Read the model definition and answer for the solid it produces. Units are mm, in the model's axes. A direction names the side the tool comes from. Give positions to 0.01 mm unless a question says otherwise; leave off trailing zeros. Order: outer loops, then holes, each group sorted by start corner. A loop starts at its lowest first (then second) coordinate and runs counter-clockwise, first axis right, second up. Notation, with made-up numbers: (45.25, 71.5) -> (104.25, 71.5) arc R19 ccw to (104.25, 81.5) -> close; hole circle Ø1 at (22, 19). An arc over 180 degrees is marked (long way). Use one line per item in the form item = value.
Autodesk Inventor part; units mm, degrees
ref_plane "YZ Plane" through (0, 0, 0) normal (1, 0, 0) x (0, 1, 0)
ref_plane "XZ Plane" through (0, 0, 0) normal (0, 1, 0) x (-1, 0, 0)
ref_plane "XY Plane" through (0, 0, 0) normal (0, 0, 1) x (1, 0, 0)
sketch "Sketch1" plane through (0, 0, 0) normal (1, 0, 0) x (0, 1, 0)
  line L0 (-7.5, 10.5) -> (7.5, 10.5)
  line L1 (7.5, 10.5) -> (7.5, -10.5)
  line L2 (7.5, -10.5) -> (-7.5, -10.5)
  line L3 (-7.5, -10.5) -> (-7.5, 10.5)
  point P0 (0, 0)
  dimension "d0" = 21
  dimension "d1" = 15
  dimension "d2" = 7.5
  dimension "d3" = 10.5
extrude "Extrusion1" add sketch "Sketch1" along normal blind 2
fillet "Fillet1" radius 1 4 edges at (1, -7.5, -10.5) (1, 7.5, -10.5) (1, 7.5, 10.5) (1, -7.5, 10.5)
sketch "Sketch2" plane through (2, 0, 0) normal (1, 0, 0) x (0, 0, -1)
  line L0 (-7.15, 4.85) -> (7.15, 4.85)
  line L1 (7.15, 4.85) -> (7.15, -4.85)
  line L2 (7.15, -4.85) -> (-7.15, -4.85)
  line L3 (-7.15, -4.85) -> (-7.15, 4.85)
  point P0 (0, 0)
  dimension "d7" = 4.85
  dimension "d8" = 9.7
  dimension "d9" = 14.3
  dimension "d10" = 7.15
ref_plane "Work Plane1" through (2, -4.85, 7.15) normal (0, -1, 0) x (1, 0, 0)
sketch "Sketch3" plane through (2, -4.85, 7.15) normal (0, -1, 0) x (1, 0, 0)
  arc A0 (3.5, -2.0473) -> (0, 0) centre (-3.3399, -9.7251) ccw
  line L0 (0, -16.65) -> (0, 2.35)
  arc A1 (3.5, -2.0473) -> (0, -14.3) centre (22.3145, -14.0479) ccw
  point P0 (-2, -7.15)
  point P1 (0, -13.7959)
  dimension "d11" = 3.5
extrude "Extrusion2" add sketch "Sketch3" against normal blind 9.7
sketch "Sketch4" plane through (0, 0, 0) normal (-1, 0, 0) x (0, 0, 1)
  line L0 (9.25, -6) -> (-9.25, -6)
  line L1 (-9.25, -6) -> (-9.25, 6)
  line L2 (-9.25, 6) -> (9.25, 6)
  line L3 (9.25, 6) -> (9.25, -6)
  line L4 (9.5, -7.5) -> (-9.5, -7.5)
  line L5 (10.5, 6.5) -> (10.5, -6.5)
  point P0 (0, 0)
  dimension "d14" = 18.5
  dimension "d15" = 12
  dimension "d16" = 1.5
  dimension "d17" = 1.25
extrude "Extrusion3" add sketch "Sketch4" along normal blind 12.3
sketch "Sketch5" plane through (-12.3, 0, 0) normal (-1, 0, 0) x (0, 0, 1)
  line L0 (9.25, -6) -> (9.25, 6)
  line L1 (-9.25, -6) -> (-9.25, 6)
  line L2 (9.25, 2.5) -> (-9.25, 2.5)
  line L3 (-9.25, 2.5) -> (-9.25, -2.5)
  line L4 (-9.25, -2.5) -> (9.25, -2.5)
  line L5 (9.25, -2.5) -> (9.25, 2.5)
  line L6 (9.25, 6) -> (-9.25, 6)
  point P0 (0, 0)
  point P1 (9.25, -2.5)
  point P2 (-9.25, 2.5)
  dimension "d20" = 5
  dimension "d21" = 3.5
extrude "Extrusion4" add sketch "Sketch5" along normal blind 6.2 contours L4 L1 L2 L0
sketch "Sketch6" plane through (-18.5, 0, 0) normal (-1, 0, 0) x (0, 0, 1)
  line L0 (9.25, 2.5) -> (-9.25, 2.5)
  line L1 (-9.25, 2.5) -> (-9.25, -2.5)
  line L2 (-9.25, -2.5) -> (9.25, -2.5)
  line L3 (9.25, -2.5) -> (9.25, 2.5)
  line L4 (9.25, 2.5) -> (8.25, 2.5)
  line L5 (8.25, 2.5) -> (8.25, -2.5)
  line L6 (8.25, -2.5) -> (9.25, -2.5)
  line L7 (9.25, -2.5) -> (9.25, 2.5)
  line L8 (7.25, -2.5) -> (0.75, -2.5)
  line L9 (0.75, -2.5) -> (0.75, 2.5)
  line L10 (0.75, 2.5) -> (7.25, 2.5)
  line L11 (7.25, 2.5) -> (7.25, -2.5)
  line L12 (-9.25, 2.5) -> (9.25, 2.5)
  line L13 (-7.25, -2.5) -> (-0.25, -2.5)
  line L14 (-0.25, -2.5) -> (-0.25, 2.5)
  line L15 (-0.25, 2.5) -> (-7.25, 2.5)
  line L16 (-7.25, 2.5) -> (-7.25, -2.5)
  line L17 (9.25, -2.5) -> (-9.25, -2.5)
  line L18 (-9.25, 2.5) -> (-8.25, 2.5)
  line L19 (-8.25, 2.5) -> (-8.25, -2.5)
  line L20 (-8.25, -2.5) -> (-9.25, -2.5)
  line L21 (-9.25, -2.5) -> (-9.25, 2.5)
  point P0 (0, 0)
  point P1 (-8.25, -2.5)
  point P2 (-0.25, -2.5)
  point P3 (7.25, 2.5)
  dimension "d24" = 1
  dimension "d25" = 1
  dimension "d26" = 1
  dimension "d27" = 1
  dimension "d28" = 1
  dimension "d29" = 6.5
extrude "Extrusion5" cut sketch "Sketch6" against normal blind 6.2 contours L3 L2 L5 L0 | L11 L2 L9 L0 | L14 L2 L16 L0 | L19 L2 L1 L0
chamfer "Chamfer1" distance 1.5 angle 45 6 edges at (-18.5, 2.5, -7.75) (-18.5, -2.5, -7.75) (-18.5, -2.5, 0.25) (-18.5, 2.5, 0.25) (-18.5, -2.5, 7.75) (-18.5, 2.5, 7.75)
sketch "Sketch7" plane through (-12.3, -2.5, -8.25) normal (0, 0, -1) x (-1, 0, 0)
  line L0 (6.2, 1.5) -> (4.7, 0)
  line L1 (6.2, 3.5) -> (6.2, 1.5)
  line L2 (4.7, 5) -> (6.2, 3.5)
  line L3 (0, 5) -> (4.7, 5)
  line L4 (0, 5) -> (0, 0)
  line L5 (4.7, 0) -> (0, 0)
  point P0 (-12.3, 2.5)
  point P1 (5.2, 2.5)
  point P2 (4.1377, 2.5)
hole "Hole1" at (-16.4377, 0, -8.25) direction (0, 0, 1) diameter 2.2 end through all
sketch "Sketch8" plane through (0, 0, 0) normal (-1, 0, 0) x (0, 0, 1)
  line L0 (-9.7, -6.55) -> (9.7, -6.55)
  line L1 (9.7, -6.55) -> (9.7, 6.55)
  line L2 (9.7, 6.55) -> (-9.7, 6.55)
  line L3 (-9.7, 6.55) -> (-9.7, -6.55)
  line L4 (-9.7, -6.55) -> (9.7, 6.55) construction
  line L5 (9.7, -6.55) -> (-9.7, 6.55) construction
  point P0 (0, 0)
  dimension "d42" = 19.4
  dimension "d43" = 13.1
properties part number "Rocker Switch" material "ABS Plastic"
Item 1: The part is cut by section D-D on x = -10.5. Give the vertices of the cut face in (y, z).
Checks:
outline = (-6, -9.25) -> (6, -9.25) -> (6, 9.25) -> (-6, 9.25) -> close
Item 2: The part is cut by section B-B on y = 0. State how many separate pieces and enclosed holes the cut face has, and give its area (3 significant figures).
Checks:
separate_pieces = 4
enclosed_holes = 0
area = 299 mm²
Item 3: Which of the six approach directions +Z, -Z, +X, -X, +Y, -Y give full straight-line access (tool end or side, diameter ignored) to faces 5 (the flat face through (3, 4.85, 3)), 6 (the flat face through (-15, 2.5, 0)), 7 (the flat face through (-15, 0, 8.25)), 8 (the flat face through (-15, -2.5, -8)), 9 (the flat face through (-15, 0, 7.25))?
Checks:
face_5 = +Z, -Z, +X, +Y
face_6 = +Z, -Z, -X, +Y
face_7 = +Z, -X, +Y, -Y
face_8 = +Z, -Z, -X, -Y
face_9 = -X, +Y, -Y
Item 4: Given pin 1 Ø1.5 at (x, y) = (-4, 1.5) entering from -Z; pin 2 Ø2 at (y, z) = (-6, -1.5) entering from -X; pin 3 Ø1 at (x, z) = (-8, -7) entering from -Y, each flat-ended and moving along its own axis, determine where each tip first touches the part or whether it passes through.
Checks:
pin_1 = -9.25
pin_2 = -12.3
pin_3 = -6
Item 5: The part is cut by section A-A on y = -4.5. Give the vertices of the cut face in (x, z), and give its area (3 significant figures).
Checks:
outline = (-12.3, -9.25) -> (0, -9.25) -> (0, -10.5) -> (2, -10.5) -> (2, -7.15) arc R22.32 cw to (5.5, 5.1) arc R10.28 ccw to (2, 7.15) -> (2, 10.5) -> (0, 10.5) -> (0, 9.25) -> (-12.3, 9.25) -> close
area = 287 mm²
Item 6: Straight lines are drawn through the part: L1, parallel to Z at x = -14, y = 0.25; L2, parallel to Y at x = -7.75, z = -1; L3, parallel to X at y = 0, z = 0.45. For each, find the intervals that lie inside material, in ascending order. Write a range as from..to.
Checks:
L1 = -8.25..-7.25, -0.25..0.75, 7.25..8.25
L2 = -6..6
L3 = -18.5..-17.54, -15.34..3.24
Item 7: The part is cut by section C-C on z = 6.5. Give the vertices of the cut face in (x, y), and give its area (3 significant figures).
Checks:
outline = (-12.3, -6) -> (0, -6) -> (0, -7.5) -> (2, -7.5) -> (2, -4.85) -> (3.49, -4.85) -> (3.49, 4.85) -> (2, 4.85) -> (2, 7.5) -> (0, 7.5) -> (0, 6) -> (-12.3, 6) -> close
area = 192 mm²
Item 8: Determine the mould class of faces 1 (the flat face through (-17.8, 1.7, 0.2)), 2 (the cylindrical face through (-15.364, -0.238, 7.757)), 3 (the cylindrical face through (-15.364, -0.238, -7.743)), 4 (the flat face through (-15, 2.5, 8)) for opening direction X: +X half, -X half, draft (parallel to the pull), parting line (faces both ways), or undercut.
Checks:
face_1 = -X half
face_2 = undercut
face_3 = undercut
face_4 = draft
